For this review, take the finished solid that the model builds, in its own axes (mm). Face numbers are marked on the shaded views. A direction names the side the tool comes from. Give positions to 0.01 mm unless a question says otherwise; leave off trailing zeros. Write each loop counter-clockwise with the first axis right and the second up, starting at its lowest first coordinate (ties: lowest second). Pieces come first, ordered by that corner, then holes. Notation, with made-up numbers: M 55.25,-0.5 L 88.25,-0.5 A31 cw 88.25,33.5 Z; hole C -38,34 d5. An arc over 180 degrees is marked long. One line per item, written item: value. Start each with the question number.
Item 1: Consider section C-C, the plane z = 25. Write out the cut boundary in (x, y).
Item 2: Mouldability with a two-part tool opening along X and no side actions: class the marked faces 3, 4 and 5 as released by +X, released by -X, zero draft, split by the parting line, or undercut.
Item 3: Clearance check with flat-ended pins moving along their axes: pin 1 Ø2 at (x, z) = (-1.5, -28) entering from -Y; pin 2 Ø5 at (x, z) = (47.5, 7.5) entering from +Y; pin 3 Ø2.5 at (y, z) = (8, -13) entering from -X; pin 4 Ø0.8 at (y, z) = (9.5, 11.5) entering from -X. State where each tip first meets the part, or that it passes through.
Item 4: Consider section D-D, the plane z = 9. Give the number of separate pieces and of enclosed holes in the cut face, and give its area (3 significant figures).
Item 5: To check wall thickness, follow probe 1 along Z at (x, y) = (0, 2.5); probe 2 along Z at (x, y) = (0.5, 7.5); probe 3 along X at (y, z) = (8.25, -16.5). State the ranges of each line that lie inside material, in increasing order.
Item 6: Tool access review of the marked faces 1 and 2: name each direction out of +Z, -Z, +X, -X, +Y, -Y from which nothing blocks a thin tool from reaching the whole face with its end or side.
Item 7: Consider section A-A, the plane x = -45. Write out the cut boundary in (y, z).
Item 8: Consider section B-B, the plane x = 12. Write out the cut boundary in (y, z).
```python
from build123d import *

# Parameters (mm, degrees)
ESQUISSE1_W               = 105
ESQUISSE1_H               = 70
ESQUISSE1_R               = 27
EXTRUSION1_DEPTH          = 10
ENL_V_START               = -8
ESQUISSE2_R               = 12.2
ENL_V_MAT_EXTRU_1_DEPTH   = 8
ESQUISSE3_R               = 2
ENL_V_MAT_EXTRU_2_DEPTH   = 66.954529791
ENL_V_MAT_EXTRU_3_DEPTH   = 1
ESQUISSE5_R               = 29
ENL_V_MAT_EXTRU_4_DEPTH   = 7
ENL_V_START_2             = -2
ESQUISSE6_R               = 29
ENL_V_MAT_EXTRU_6_DEPTH   = 2
ENL_V_MAT_EXTRU_7_REACH   = 67.955
ESQUISSE7_W               = 8
ESQUISSE7_H               = 24
ENL_V_MAT_EXTRU_8_DEPTH   = 3
TROU_TARAUD_M4X0_71_D     = 3.3
TROU_TARAUD_M4X0_71_DEPTH = 12.1
TROU_TARAUD_M4X0_71_TIP   = 0.991420021
TROU_TARAUD_M4X0_72_D     = 3.3


with BuildPart() as part:
    # Esquisse1 → Extrusion1 (new body)
    with BuildSketch(Plane(origin=(0, 0, 0), x_dir=(1, 0, 0), z_dir=(0, 1, 0))):
        with Locations((2.5, 0)):
            Rectangle(ESQUISSE1_W, ESQUISSE1_H)
        with Locations(Location((0, 0, 0), (0, 0, 270))):
            Circle(ESQUISSE1_R, mode=Mode.SUBTRACT)
    extrude(amount=EXTRUSION1_DEPTH)

    # Esquisse2 → Enlèv. mat.-Extru.1 (cut)
    with BuildSketch(Plane(origin=(0, 10, 0), x_dir=(-1, 0, 0), z_dir=(0, 1, 0)).offset(ENL_V_START)):
        with Locations(Location((-40, -20, 0), (0, 0, 90))):
            Circle(ESQUISSE2_R)
    extrude(amount=ENL_V_MAT_EXTRU_1_DEPTH, mode=Mode.SUBTRACT)

    # Esquisse3 → Enlèv. mat.-Extru.2 (cut, through all)
    with BuildSketch(Plane(origin=(0, 0, 0), x_dir=(1, 0, 0), z_dir=(0, 1, 0))):
        with Locations(Location((45, -9, 0), (0, 0, 270))):
            Circle(ESQUISSE3_R)
        with Locations(Location((-45, -9, 0), (0, 0, 270))):
            Circle(ESQUISSE3_R)
        with BuildLine():
            Line((32.2, 18.5), (55, 18.5))
            Line((55, 18.5), (55, 21.5))
            Line((55, 21.5), (32.2, 21.5))
            ThreePointArc((32.2, 21.5), (30.7, 20), (32.2, 18.5))
        make_face()
    extrude(amount=ENL_V_MAT_EXTRU_2_DEPTH, mode=Mode.SUBTRACT)

    # Esquisse4 → Enlèv. mat.-Extru.3 (cut)
    with BuildSketch(Plane(origin=(0, 10, 0), x_dir=(-1, 0, 0), z_dir=(0, 1, 0))):
        with BuildLine():
            Line((-50, 14), (-40, 14))
            ThreePointArc((-40, 14), (-38.939339828, 13.560660172), (-38.5, 12.5))
            Line((-38.5, 12.5), (-38.5, 5.5))
            ThreePointArc((-38.5, 5.5), (-38.939339828, 4.439339828), (-40, 4))
            Line((-40, 4), (-50, 4))
            ThreePointArc((-50, 4), (-51.060660172, 4.439339828), (-51.5, 5.5))
            Line((-51.5, 5.5), (-51.5, 12.5))
            ThreePointArc((-51.5, 12.5), (-51.060660172, 13.560660172), (-50, 14))
        make_face()
        with BuildLine():
            Line((50, 14), (43, 14))
            ThreePointArc((43, 14), (41.5, 15.5), (40, 14))
            Line((40, 14), (40, 4))
            ThreePointArc((40, 4), (41.5, 2.5), (43, 4))
            Line((43, 4), (50, 4))
            Line((50, 4), (50, 14))
        make_face()
    extrude(amount=-ENL_V_MAT_EXTRU_3_DEPTH, mode=Mode.SUBTRACT)

    # Esquisse5 → Enlèv. mat.-Extru.4 (cut)
    with BuildSketch(Plane(origin=(0, 0, 0), x_dir=(1, 0, 0), z_dir=(0, 1, 0))):
        Circle(ESQUISSE5_R)
    extrude(amount=ENL_V_MAT_EXTRU_4_DEPTH, mode=Mode.SUBTRACT)

    # Esquisse6 → Enlèv. mat.-Extru.6 (cut)
    with BuildSketch(Plane(origin=(0, 10, 0), x_dir=(-1, 0, 0), z_dir=(0, 1, 0)).offset(ENL_V_START_2)):
        with Locations(Location((0, 0, 0), (0, 0, 180))):
            Circle(ESQUISSE6_R)
    extrude(amount=ENL_V_MAT_EXTRU_6_DEPTH, mode=Mode.SUBTRACT)

    # Esquisse7 → Enlèv. mat.-Extru.7 (cut, up to next)
    with BuildSketch(Plane(origin=(0, 0, 0), x_dir=(1, 0, 0), z_dir=(0, 1, 0)), mode=Mode.PRIVATE) as enl_v_mat_extru_7_sk1:
        with Locations((-46, 11)):
            Rectangle(ESQUISSE7_W, ESQUISSE7_H)
    enl_v_mat_extru_7_tool1 = extrude(enl_v_mat_extru_7_sk1.sketch, amount=ENL_V_MAT_EXTRU_7_REACH, mode=Mode.PRIVATE) & part.part
    add(enl_v_mat_extru_7_tool1.solids().sort_by_distance((-46, 0, -11))[0], mode=Mode.SUBTRACT)

    # Esquisse8 → Enlèv. mat.-Extru.8 (cut)
    with BuildSketch(Plane(origin=(0, 10, 0), x_dir=(-1, 0, 0), z_dir=(0, 1, 0))):
        with BuildLine():
            Line((50, -23), (38, -23))
            ThreePointArc((38, -23), (36.939339828, -22.560660172), (36.5, -21.5))
            Line((36.5, -21.5), (36.5, -0.5))
            ThreePointArc((36.5, -0.5), (36.939339828, 0.560660172), (38, 1))
            Line((38, 1), (50, 1))
            Line((50, 1), (50, -23))
        make_face()
    extrude(amount=-ENL_V_MAT_EXTRU_8_DEPTH, mode=Mode.SUBTRACT)

    # Trou taraudé M4x0.71
    with Locations(Plane.ZY.offset(42)):
        with Locations((-11, 3.5)):
            Hole(TROU_TARAUD_M4X0_71_D / 2, depth=TROU_TARAUD_M4X0_71_DEPTH)
            with Locations((0, 0, -(TROU_TARAUD_M4X0_71_DEPTH + TROU_TARAUD_M4X0_71_TIP / 2))):  # 118° drill point
                Cone(0, TROU_TARAUD_M4X0_71_D / 2, TROU_TARAUD_M4X0_71_TIP, mode=Mode.SUBTRACT)

    # Trou taraudé M4x0.72 (through all)
    with Locations(Plane.XZ):
        with Locations((-45, -30), (50, 30)):
            Hole(TROU_TARAUD_M4X0_72_D / 2)


solid = part.part
```
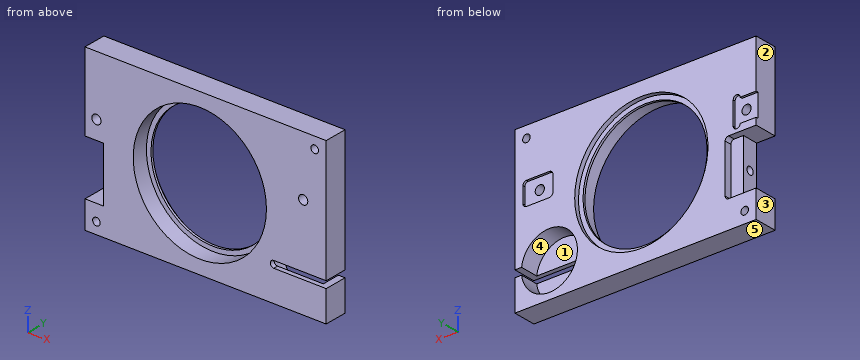
Model answer:
1. outline: M -50,0 L -14.7,0 L -14.7,7 L -10.2,7 L -10.2,8 L -14.7,8 L -14.7,10 L -50,10 Z; M 10.2,7 L 14.7,7 L 14.7,0 L 55,0 L 55,10 L 14.7,10 L 14.7,8 L 10.2,8 Z
2. face 3: released by -X
2. face 4: undercut
2. face 5: zero draft
3. pin 1: stops at y = 0
3. pin 2: stops at y = 9
3. pin 3: stops at x = -42
3. pin 4: stops at x = -40
4. separate pieces: 4
4. enclosed holes: 0
4. area: 408 mm2
5. probe 1: z = -35 to -29, 29 to 35
5. probe 2: z = -35 to -27, 27 to 35
5. probe 3: x = -36.5 to -23.85, 23.85 to 28.31, 51.69 to 55
6. face 1: +Y
6. face 2: +Z, -Z, -X, +Y, -Y
7. outline: M 0,-35 L 10,-35 L 10,-31.65 L 0,-31.65 Z; M 0,-28.35 L 10,-28.35 L 10,-23 L 0,-23 Z; M 0,1 L 10,1 L 10,4 L 9,4 L 9,7 L 0,7 Z; M 0,11 L 9,11 L 9,14 L 10,14 L 10,35 L 0,35 Z
8. outline: M 0,-35 L 10,-35 L 10,-26.4 L 8,-26.4 L 8,-24.19 L 7,-24.19 L 7,-26.4 L 0,-26.4 Z; M 0,26.4 L 7,26.4 L 7,24.19 L 8,24.19 L 8,26.4 L 10,26.4 L 10,35 L 0,35 Z
